Can you work these out from the drawing? Everything is in mm from the part's minimum corner. Round coordinates to 2 decimals unless told otherwise and drop trailing zeros. Order: outer loops, then holes, each group sorted by start corner. A loop starts at its lowest first (then second) coordinate and runs counter-clockwise, first axis right, second up. Notation, with made-up numbers: M 79,79 L 129,79 A20 cw 129,109 Z; hole C 71.5,59 d6. An arc over 180 degrees is marked long. Write each question's results on one line, items separated by ' | '. Start each with the question number.
1. I'm going to push a flat-ended pin straight in: pin 1 (0.5 mm diameter, centred on y = 4, z = 0.5, fed in from -X). Where does the tip first touch, or does it pass through?
2. Please list where these lines run through material, in increasing order: L1, parallel to Y at x = 14, z = 0.6; L2, parallel to Y at x = 11.75, z = 0.3; L3, parallel to X at y = 9, z = 0.45.
3. Suppose I cut it at A-A on x = 14. Write out the boundary of the cut face in (y, z).
4. Suppose I cut it at B-B on z = 0.15. Write out the boundary of the cut face in (x, y), and give its area (3 significant figures).
5. Suppose I cut it at D-D on x = 9.25. Write out the boundary of the cut face in (y, z).
6. Suppose I cut it at C-C on y = 19. Write out the boundary of the cut face in (x, z).
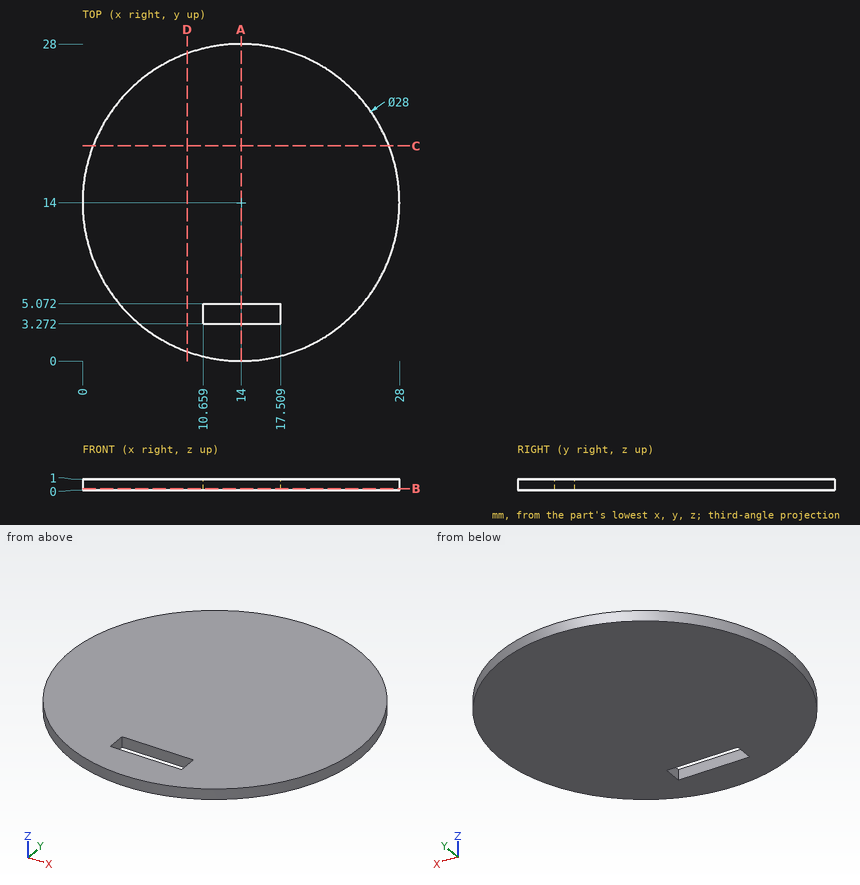
Filled sheet:
1) pin 1: stops at x = 3.95
2) L1: y = 0 to 3.27, 5.07 to 28 | L2: y = 0.18 to 3.27, 5.07 to 27.82 | L3: x = 0.92 to 27.08
3) outline: M 0,0 L 3.27,0 L 3.27,1 L 0,1 Z; M 5.07,0 L 28,0 L 28,1 L 5.07,1 Z
4) outline: C 14,14 d28; hole M 10.66,3.27 L 17.51,3.27 L 17.51,5.07 L 10.66,5.07 Z | area: 603 mm^2
5) outline: M 0.83,0 L 27.17,0 L 27.17,1 L 0.83,1 Z
6) outline: M 0.92,0 L 27.08,0 L 27.08,1 L 0.92,1 Z
